Autodesk Inventor part; units mm, degrees
ref_plane "YZ Plane" through (0, 0, 0) normal (1, 0, 0) x (0, 1, 0)
ref_plane "XZ Plane" through (0, 0, 0) normal (0, 1, 0) x (-1, 0, 0)
ref_plane "XY Plane" through (0, 0, 0) normal (0, 0, 1) x (1, 0, 0)
sketch "Sketch1" plane through (0, 0, 0) normal (1, 0, 0) x (0, 1, 0)
  line L0 (0, 0) -> (0, -63.5)
  line L1 (0, -63.5) -> (63.5, -63.5)
  line L2 (63.5, -63.5) -> (63.5, -60.96)
  line L3 (0, 0) -> (2.54, 0)
  line L4 (2.54, 0) -> (2.54, -60.96)
  line L5 (2.54, -60.96) -> (63.5, -60.96)
  dimension "d0" = 63.5
  dimension "d1" = 63.5
  dimension "d2" = 2.54
  dimension "d3" = 2.54
extrude "Extrusion1" add sketch "Sketch1" along normal blind 15.875
sketch "Sketch2" plane through (0, 2.54, 0) normal (0, 1, 0) x (1, 0, 0)
  circle A0 centre (6.35, 7.9375) radius 3.175
  circle A1 centre (9.525, 49.2125) radius 3.175
  point P0 (0, 0)
  dimension "d6" = 6.35
  dimension "d7" = 6.35
extrude "Extrusion2" cut sketch "Sketch2" against normal through all contours A1
extrude "Extrusion3" cut sketch "Sketch2" against normal through all contours A0
sketch "Sketch3" plane through (0, 2.54, -60.96) normal (0, 0, 1) x (1, 0, 0)
  line L0 (15.875, 60.96) -> (15.875, 53.0225)
  line L1 (15.875, 53.0225) -> (9.525, 53.0225)
  line L2 (15.875, 53.0225) -> (15.875, 11.7475)
  line L3 (15.875, 11.7475) -> (6.35, 11.7475)
  circle A0 centre (6.35, 11.7475) radius 3.175
  circle A1 centre (9.525, 53.0225) radius 3.175
  point P0 (0, -2.54)
  dimension "d12" = 6.35
  dimension "d13" = 6.35
  dimension "d14" = 6.35
  dimension "d15" = 7.9375
  dimension "d16" = 41.275
  dimension "d17" = 9.525
extrude "Extrusion4" cut sketch "Sketch3" against normal through all contours A0
extrude "Extrusion5" cut sketch "Sketch3" against normal through all contours A1
properties part number "Plywood Pickle Mount Corner Bracket"
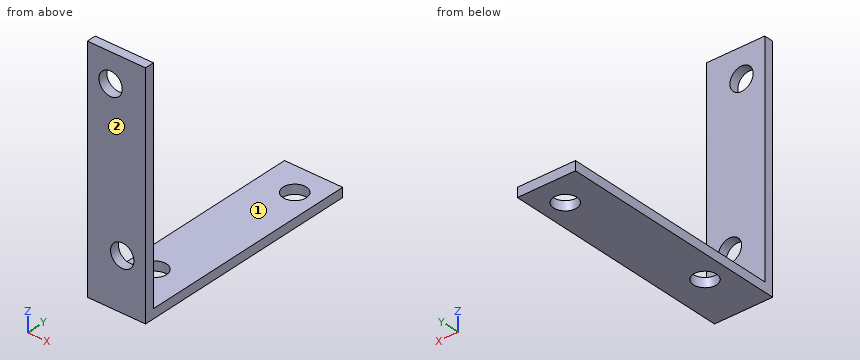
For this review, take the finished solid that the model builds, in its own axes (mm). Face numbers are marked on the shaded views. A direction names the side the tool comes from. Give positions to 0.01 mm unless a question says otherwise; leave off trailing zeros. Loops run counter-clockwise (first coordinate to the right, second up) from the corner with the lowest first, then second, coordinate; pieces in that order, holes last. Notation, with made-up numbers: (-16.75, -37) - (3.25, -37) arc R36 cw to (3.25, -2) - close; hole circle Ø11 at (-36, 51). An arc over 180 degrees is marked (long way). Write each question's results on one line, items separated by ' | '.
(1) For pin 1 Ø8 at (x, z) = (7.5, -55.5) entering from +Y; pin 2 Ø1.5 at (x, y) = (10.5, 55) entering from -Z; pin 3 Ø7.5 at (x, y) = (9.52, 55.56) entering from -Z; pin 4 Ø8 at (x, y) = (4, 47) entering from +Z, all flat-tipped, find the tip position at first contact; note any pin that passes through.
Conclusion:
pin 1: y = 2.54 | pin 2: through | pin 3: z = -63.5 | pin 4: z = -60.96
(2) For line 1 along Y through (x, z) = (9, -59); line 2 along Z through (x, y) = (14.25, 19.5), list the stretches that pass through material, from the lowest coordinate up.
Conclusion:
line 1: 0 to 2.54 | line 2: -63.5 to -60.96
(3) Take a section at D-D (z = -19.5). Give the boundary of the cut face in (x, y) (3 decimals), then the cut area to 3 significant figures.
Conclusion:
outline: (0, 0) - (15.875, 0) - (15.875, 2.54) - (0, 2.54) - close | area: 40.3 mm^2
(4) For the marked faces 1 and 2, list the 3-axis set-ups (+Z, -Z, +X, -X, +Y, -Y) from which the entire face can be reached by the end or side of a thin tool; tool diameter is ignored.
Conclusion:
face 1: +Z, +X, -X, +Y | face 2: +Z, -Z, +X, -X, -Y
(5) Take a section at B-B (x = 4.75). Give the boundary of the cut face in (y, z).
Conclusion:
outline: (0, -63.5) - (11.55, -63.5) - (11.55, -60.96) - (2.54, -60.96) - (2.54, -10.68) - (0, -10.68) - close; (0, -5.2) - (2.54, -5.2) - (2.54, 0) - (0, 0) - close; (17.03, -63.5) - (63.5, -63.5) - (63.5, -60.96) - (17.03, -60.96) - close
(6) Take a section at A-A (z = -50.5). Give the boundary of the cut face in (x, y) (3 decimals).
Conclusion:
outline: (0, 0) - (6.623, 0) - (6.623, 2.54) - (0, 2.54) - close; (12.427, 0) - (15.875, 0) - (15.875, 2.54) - (12.427, 2.54) - close
(7) Take a section at C-C (x = 8.5). Give the boundary of the cut face in (y, z).
Conclusion:
outline: (0, -63.5) - (11.95, -63.5) - (11.95, -60.96) - (2.54, -60.96) - (2.54, -52.22) - (0, -52.22) - close; (0, -46.21) - (2.54, -46.21) - (2.54, -10.27) - (0, -10.27) - close; (0, -5.6) - (2.54, -5.6) - (2.54, 0) - (0, 0) - close; (16.62, -63.5) - (52.56, -63.5) - (52.56, -60.96) - (16.62, -60.96) - close; (58.57, -63.5) - (63.5, -63.5) - (63.5, -60.96) - (58.57, -60.96) - close
